Read the model definition and answer for the solid it produces. Units are mm, in the model's axes. Face numbers are marked on the shaded views. A direction names the side the tool comes from. Coordinates: 2 decimals unless noted, no trailing zeros. Write each loop counter-clockwise with the first axis right and the second up, starting at its lowest first coordinate (ties: lowest second). Pieces come first, ordered by that corner, then holes. Notation, with made-up numbers: (-6.5, 88.5) -> (25.5, 88.5) arc R21 cw to (25.5, 116.5) -> close; hole circle Ø2 at (76, -8). An arc over 180 degrees is marked (long way). Answer in a Markdown table with one row per item. Add a question column.
Item 1: Section C-C on z = -58.5 is taken. Write down the section's boundary in (x, y).
Item 2: For a pull along Z with two mould halves and no side action, classify the marked faces 1, 2, 3 and 4 as +Z half, -Z half, draft (parallel to the pull), parting line (faces both ways), or undercut.
Item 3: Which of the six approach directions +Z, -Z, +X, -X, +Y, -Y give full straight-line access (tool end or side, diameter ignored) to the marked faces 5, 6 and 7?
Item 4: Section B-B on x = 50 is taken. Write down the section's boundary in (y, z).
Item 5: Given pin 1 Ø8 at (x, z) = (12.5, -27.5) entering from -Y, flat-ended and moving along its own axis, determine where the tip first touches the part or whether it passes through.
Item 6: Section A-A on y = -50 is taken. Write down the section's boundary in (x, z), then the cut area to 3 significant figures.
Item 7: Straight lines are drawn through the part: line 1 (X direction, y = -85, z = -63.5); line 2 (Z direction, x = 39.5, y = -6.5); line 3 (Y direction, x = -51.5, z = 32). For each, find the intervals that lie inside material, in ascending order. Write a range as from..to.
Item 8: Section D-D on z = -42 is taken. Write down the section's boundary in (x, y).
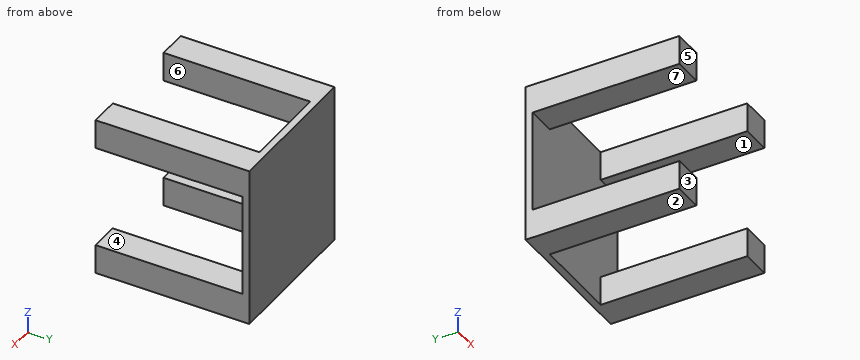
```python
from build123d import *

# Parameters (mm, degrees)
F0_W     = 127
F0_H     = 139.7
F1_DEPTH = 6.096
F2_W     = 25.4
F2_H     = 25.4
F3_DEPTH = 127
F4_DEPTH = 127
F5_DEPTH = 127
F6_DEPTH = 127


with BuildPart() as f1:
    # F0 (on Front) → F1 (new body)
    with BuildSketch(Plane.XZ):
        Rectangle(F0_W, F0_H)
    extrude(amount=F1_DEPTH)

    # F2 (on face) → F3 (join)
    with BuildSketch(Plane.XZ.offset(6.096)):
        with Locations((-50.8, 57.15)):
            Rectangle(F2_W, F2_H)
    extrude(amount=F3_DEPTH)

    # F2 (on face) → F4 (join)
    with BuildSketch(Plane.XZ.offset(6.096)):
        with Locations((-50.8, -57.15)):
            Rectangle(F2_W, F2_H)
    extrude(amount=F4_DEPTH)

    # F2 (on face) → F5 (join)
    with BuildSketch(Plane.XZ.offset(6.096)):
        with Locations((50.8, 57.15)):
            Rectangle(F2_W, F2_H)
    extrude(amount=F5_DEPTH)

    # F2 (on face) → F6 (join)
    with BuildSketch(Plane.XZ.offset(6.096)):
        with Locations((50.8, -57.15)):
            Rectangle(F2_W, F2_H)
    extrude(amount=F6_DEPTH)


solid = f1.part
```
Results below:
| question | item | result |
|---|---|---|
| 1 | outline | (-63.5, -133.1) -> (-38.1, -133.1) -> (-38.1, -6.1) -> (38.1, -6.1) -> (38.1, -133.1) -> (63.5, -133.1) -> (63.5, 0) -> (-63.5, 0) -> close |
| 2 | face 1 | undercut |
| 2 | face 2 | -Z half |
| 2 | face 3 | draft |
| 2 | face 4 | undercut |
| 3 | face 5 | +Z, -Z, +X, -X, -Y |
| 3 | face 6 | +Z, -Z, -Y |
| 3 | face 7 | +X, -X, -Y |
| 4 | outline | (-133.1, -69.85) -> (0, -69.85) -> (0, 69.85) -> (-133.1, 69.85) -> (-133.1, 44.45) -> (-6.1, 44.45) -> (-6.1, -44.45) -> (-133.1, -44.45) -> close |
| 5 | pin 1 | stops at y = -6.1 |
| 6 | outline | (-63.5, -69.85) -> (-38.1, -69.85) -> (-38.1, -44.45) -> (-63.5, -44.45) -> close; (-63.5, 44.45) -> (-38.1, 44.45) -> (-38.1, 69.85) -> (-63.5, 69.85) -> close; (38.1, -69.85) -> (63.5, -69.85) -> (63.5, -44.45) -> (38.1, -44.45) -> close; (38.1, 44.45) -> (63.5, 44.45) -> (63.5, 69.85) -> (38.1, 69.85) -> close |
| 6 | area | 2,580 mm2 |
| 7 | line 1 | x = -63.5..-38.1, 38.1..63.5 |
| 7 | line 2 | z = -69.85..-44.45, 44.45..69.85 |
| 7 | line 3 | y = -6.1..0 |
| 8 | outline | (-63.5, -6.1) -> (63.5, -6.1) -> (63.5, 0) -> (-63.5, 0) -> close |
